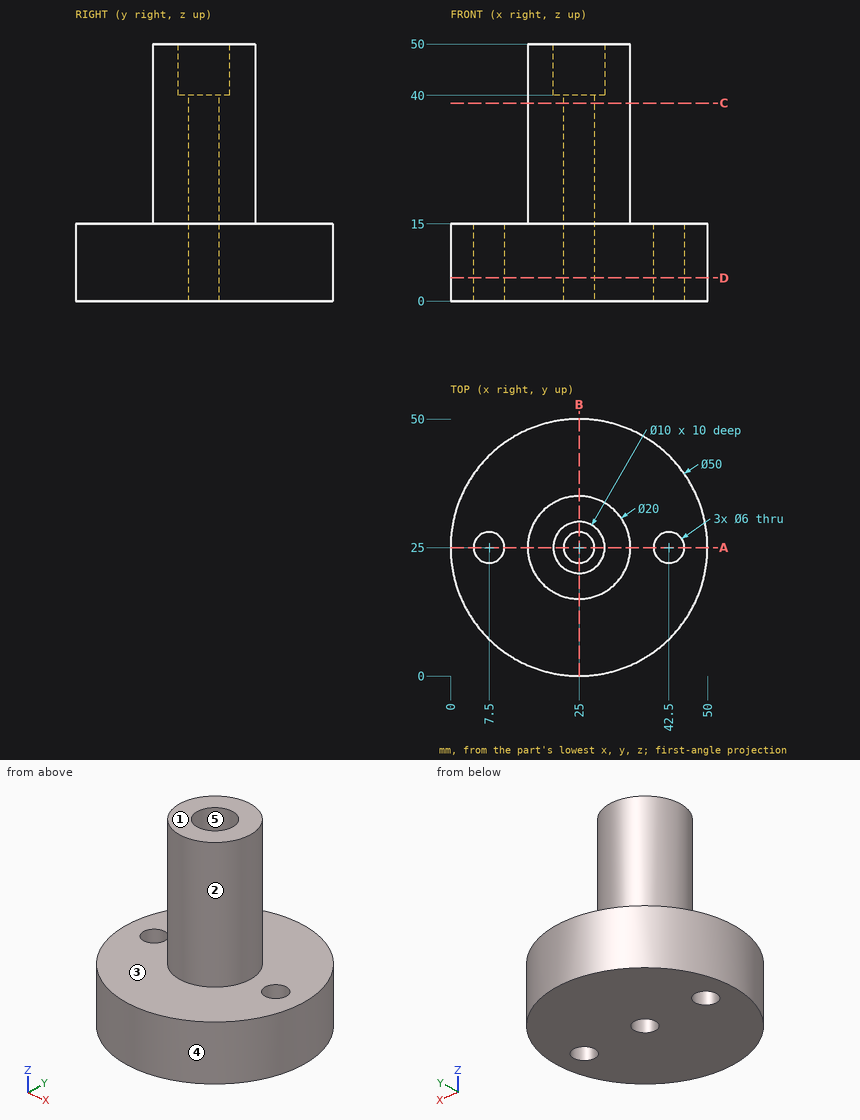
Here's the drawing with two shaded views (mm, measured from the low corner). I have some questions. A direction names the side the tool comes from. Coordinates: 2 decimals unless noted, no trailing zeros. Write each loop counter-clockwise with the first axis right and the second up, starting at its lowest first coordinate (ties: lowest second). Pieces come first, ordered by that corner, then holes. Notation, with made-up numbers: (73.5, -18) - (97.5, -18) arc R18 ccw to (97.5, 3) - close; hole circle Ø3 at (7, 77.25). An arc over 180 degrees is marked (long way). Return JSON: item names as keys, results as strings.
Q1. If we section it at C-C (z = 38.5): Please give me the cut outline in (x, y).
Computed values:
{"outline": "circle Ø20 at (25, 25); hole circle Ø6 at (25, 25)"}
Q2. If we section it at B-B (x = 25): Please give me the cut outline in (y, z), then the cut area to 3 significant figures.
Computed values:
{"outline": "(0, 0) - (22, 0) - (22, 40) - (20, 40) - (20, 50) - (15, 50) - (15, 15) - (0, 15) - close; (28, 0) - (50, 0) - (50, 15) - (35, 15) - (35, 50) - (30, 50) - (30, 40) - (28, 40) - close", "area": "1,110 mm2"}
Q3. Please list where these lines run through material, in increasing order: L1, parallel to Y at x = 25, z = 22; L2, parallel to Z at x = 27, y = 37; L3, parallel to Y at x = 24, z = 10.5. Write a range as from..to.
Computed values:
{"L1": "y = 15..22, 28..35", "L2": "z = 0..15", "L3": "y = 0.02..22.17, 27.83..49.98"}
Q4. If we section it at D-D (z = 4.5): Please give me the cut outline in (x, y).
Computed values:
{"outline": "circle Ø50 at (25, 25); hole circle Ø6 at (7.5, 25); hole circle Ø6 at (25, 25); hole circle Ø6 at (42.5, 25)"}
Q5. I'm going to push flat-ended pins straight in: pin 1 Ø8 at (x, y) = (42.5, 25) entering from -Z; pin 2 Ø8 at (y, z) = (20.5, 6) entering from +X (3 decimals); pin 3 Ø1.5 at (y, z) = (27.5, 43.5) entering from -X; pin 4 Ø12 at (y, z) = (13.5, 30.5) entering from -X. Where does each tip first touch, or does it pass through?
Computed values:
{"pin 1": "stops at z = 0", "pin 2": "stops at x = 49.995", "pin 3": "stops at x = 15.15", "pin 4": "stops at x = 16.65"}
Q6. On a 3-axis mill with a long thin cutter (end or side, diameter ignored), from which of +Z, -Z, +X, -X, +Y, -Y can I reach the whole of each face in a straight line? I mean the marked faces 1 and 2. Say none if no direction works.
Computed values:
{"face 1": "+Z, +X, -X, +Y, -Y", "face 2": "+Z"}
Q7. If we section it at A-A (y = 25): Please give me the cut outline in (x, z).
Computed values:
{"outline": "(0, 0) - (4.5, 0) - (4.5, 15) - (0, 15) - close; (10.5, 0) - (22, 0) - (22, 40) - (20, 40) - (20, 50) - (15, 50) - (15, 15) - (10.5, 15) - close; (28, 0) - (39.5, 0) - (39.5, 15) - (35, 15) - (35, 50) - (30, 50) - (30, 40) - (28, 40) - close; (45.5, 0) - (50, 0) - (50, 15) - (45.5, 15) - close"}
Q8. Thinking about a two-plate mould opening in X: for the marked faces 3, 4 and 5, which applies, +X half, -X half, draft (parallel to the pull), parting line (faces both ways), or undercut?
Computed values:
{"face 3": "draft", "face 4": "parting line", "face 5": "undercut"}
